from build123d import *

# Parameters (mm, degrees)
SKETCH_1_R          = 3
SKETCH_1_W          = 4
SKETCH_1_H          = 6
EXTRUDE_1_DEPTH     = 3
SKETCH_1_4_R        = 2
SKETCH_1_4_W        = 4
SKETCH_1_4_H        = 4
EXTRUDE_2_DEPTH     = 5
SKETCH_1_5_R        = 1.5
CUT_EXTRUDE_1_DEPTH = 6


with BuildPart() as part:
    # Sketch 1 → Extrude 1 (new body)
    with BuildSketch(Plane.XY):
        with Locations((-2, 0)):
            Circle(SKETCH_1_R)
        with Locations((2, 0)):
            Circle(SKETCH_1_R)
        Rectangle(SKETCH_1_W, SKETCH_1_H)
    extrude(amount=EXTRUDE_1_DEPTH)

    # Sketch 1_4 → Extrude 2 (add)
    with BuildSketch(Plane.XY):
        with Locations((-2, 0)):
            Circle(SKETCH_1_4_R)
        with Locations((2, 0)):
            Circle(SKETCH_1_4_R)
        Rectangle(SKETCH_1_4_W, SKETCH_1_4_H)
    extrude(amount=EXTRUDE_2_DEPTH)

    # Sketch 1_5 → Cut-Extrude 1 (cut, through all)
    with BuildSketch(Plane.XY):
        with Locations((-2, 0)):
            Circle(SKETCH_1_5_R)
        with Locations((2, 0)):
            Circle(SKETCH_1_5_R)
    extrude(amount=CUT_EXTRUDE_1_DEPTH, mode=Mode.SUBTRACT)


solid = part.part
Read the model definition and answer for the solid it produces. Units are mm, in the model's axes. A direction names the side the tool comes from. Round coordinates to 2 decimals unless told otherwise and drop trailing zeros. Loops run counter-clockwise (first coordinate to the right, second up) from the corner with the lowest first, then second, coordinate; pieces in that order, holes last.
Q1. Which of the six approach directions +Z, -Z, +X, -X, +Y, -Y give full straight-line access (tool end or side, diameter ignored) to faces 1 (the face through (0, 2, 4)), 2 (the face through (-0.1, 2.7, 3)), 3 (the face through (0, -2, 4))?
Q2. Determine the mould class of faces 4 (the face through (-4, 0, 4)), 5 (the face through (0.5, 0.07, 2.46)), 6 (the face through (5, 0, 1)) for opening direction X: released by +X, released by -X, zero draft, split by the parting line, or undercut.
Q3. Section D-D on z = 0.35 is taken. Write down the section's boundary in (x, y).
Q4. Consider probe 1 along X at (y, z) = (0, 2.05); probe 2 along X at (y, z) = (0, 3.6); probe 3 along Y at (x, z) = (-2, 3.95). Determine where each line is inside the solid, lowest interval first.
Q5. Section C-C on y = 1.25 is taken. Write down the section's boundary in (x, z).
Q6. Section B-B on x = 2.75 is taken. Write down the section's boundary in (y, z), and give its area (3 significant figures).
Q7. Each of these flat-tipped pins is pushed along its axis until it touches: pin 1 (0.6 mm diameter, centred on x = -0.5, z = 4.5, fed in from +Y); pin 2 (0.6 mm diameter, centred on x = 0.5, z = 4, fed in from -Y); pin 3 (2 mm diameter, centred on y = 2.5, z = 4.5, fed in from -X). Where does it stop, or does it pass through?
Q8. Section A-A on z = 3.3 is taken. Write down the section's boundary in (x, y).
Output:
1. face 1: +Z, +X, -X, +Y
1. face 2: +Z
1. face 3: +Z, +X, -X, -Y
2. face 4: released by -X
2. face 5: undercut
2. face 6: released by +X
3. outline: (-2, -3) - (2, -3) arc R3 ccw to (2, 3) - (-2, 3) arc R3 ccw to start; hole circle Ø3 at (-2, 0); hole circle Ø3 at (2, 0)
4. probe 1: x = -5 to -3.5, -0.5 to 0.5, 3.5 to 5
4. probe 2: x = -4 to -3.5, -0.5 to 0.5, 3.5 to 4
4. probe 3: y = -2 to -1.5, 1.5 to 2
5. outline: (-4.73, 0) - (-2.83, 0) - (-2.83, 5) - (-3.56, 5) - (-3.56, 3) - (-4.73, 3) - close; (-1.17, 0) - (1.17, 0) - (1.17, 5) - (-1.17, 5) - close; (2.83, 0) - (4.73, 0) - (4.73, 3) - (3.56, 3) - (3.56, 5) - (2.83, 5) - close
6. outline: (-2.9, 0) - (-1.3, 0) - (-1.3, 5) - (-1.85, 5) - (-1.85, 3) - (-2.9, 3) - close; (1.3, 0) - (2.9, 0) - (2.9, 3) - (1.85, 3) - (1.85, 5) - (1.3, 5) - close
6. area: 11.9 mm2
7. pin 1: stops at y = 2
7. pin 2: stops at y = -2
7. pin 3: stops at x = -3.32
8. outline: (-2, -2) - (2, -2) arc R2 ccw to (2, 2) - (-2, 2) arc R2 ccw to start; hole circle Ø3 at (-2, 0); hole circle Ø3 at (2, 0)
